```python
from build123d import *

# Parameters (mm, degrees)
DOGPOINT_DEPTH = 5.24


with BuildPart() as part:
    # BodySke → BaseBody (revolve)
    with BuildSketch(Plane.XY, mode=Mode.PRIVATE) as basebody_sk:
        with BuildLine():
            Line((19.5, 6.107179677), (16.221539031, 8))
            Line((16.221539031, 8), (2, 8))
            Line((2, 8), (0, 6))
            Line((0, 6), (0, 0))
            Line((0, 0), (122.4, 0))
            Line((122.4, 0), (122.4, 6))
            Line((122.4, 6), (120.4, 8))
            Line((120.4, 8), (105.964101615, 8))
            Line((105.964101615, 8), (102.685640646, 6.107179677))
            ThreePointArc((102.685640646, 6.107179677), (102.492695882, 6.027259339), (102.285640646, 6))
            Line((102.285640646, 6), (100.8, 6))
            ThreePointArc((100.8, 6), (100.234314575, 6.234314575), (100, 6.8))
            Line((100, 6.8), (100, 8))
            Line((100, 8), (22.4, 8))
            Line((22.4, 8), (22.4, 6.8))
            ThreePointArc((22.4, 6.8), (22.165685425, 6.234314575), (21.6, 6))
            Line((21.6, 6), (19.9, 6))
            ThreePointArc((19.9, 6), (19.692944764, 6.027259339), (19.5, 6.107179677))
        make_face()
    revolve(basebody_sk.sketch.rotate(Axis((-3.175, 0, 0), (1, 0, 0)), 90), axis=Axis((-3.175, 0, 0), (1, 0, 0)))

    # DogPointSke → DogPoint (add)
    with BuildSketch(Plane(origin=(122.4, 0, 0), x_dir=(0, 0, -1), z_dir=(1, 0, 0))):
        with BuildLine():
            Line((-5, 3.31662479), (-5, -3.31662479))
            ThreePointArc((-5, -3.31662479), (0, -6), (5, -3.31662479))
            Line((5, -3.31662479), (5, 3.31662479))
            ThreePointArc((5, 3.31662479), (0, 6), (-5, 3.31662479))
        make_face()
    extrude(amount=DOGPOINT_DEPTH)


solid = part.part
```
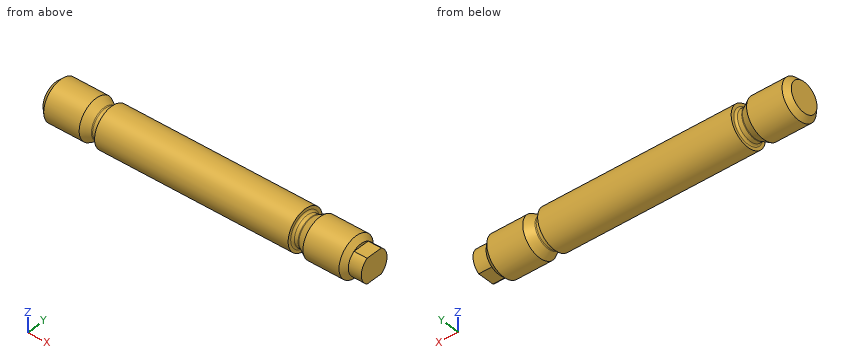
Here's how the part is built. I have some questions about the finished solid (model axes, mm). Coordinates: 2 decimals unless noted, no trailing zeros. Write each loop counter-clockwise with the first axis right and the second up, starting at its lowest first coordinate (ties: lowest second). Pieces come first, ordered by that corner, then holes. Notation, with made-up numbers: (41.25, 1) -> (63.25, 1) arc R18 cw to (63.25, 27) -> close; hole circle Ø4 at (51.5, 73). An arc over 180 degrees is marked (long way). Use a Markdown table: item, result. Add a question column.
(1) Please list where these lines run through material, in increasing order: line 1 (X direction, y = 4.25, z = -5); line 2 (X direction, y = -4.5, z = -5.75); line 3 (Z direction, x = 41, y = 6.25).
(2) If we section it at B-B, the plane x = 48: Write out the boundary of the cut face in (y, z).
(3) I'm going to push flat-ended pins straight in: P1, Ø8, axis at x = 52.5, y = 6.5, coming from the -Z side; P2, Ø1, axis at x = 48, z = 1, coming from the +Y side; P3, Ø1.6, axis at x = 124.5, y = 0, coming from the +Z side. Where does each tip first touch, or does it pass through?
Outcome:
| question | item | result |
|---|---|---|
| 1 | line 1 | x = 0.56 to 18.71, 22.36 to 100.04, 103.47 to 121.84 |
| 1 | line 2 | x = 1.3 to 17.43, 22.4 to 100, 104.75 to 121.1 |
| 1 | line 3 | z = -4.99 to 4.99 |
| 2 | outline | circle Ø16 at (0, 0) |
| 3 | P1 | stops at z = -7.6 |
| 3 | P2 | stops at y = 7.98 |
| 3 | P3 | stops at z = 5 |
